Source: CAD feature listing. Evaluate the final solid. Frame: model axes, mm. A direction names the side the tool comes from. Give positions to 0.01 mm unless a question says otherwise; leave off trailing zeros. Write each loop counter-clockwise with the first axis right and the second up, starting at its lowest first coordinate (ties: lowest second). Pieces come first, ordered by that corner, then holes. Notation, with made-up numbers: (7.5, 18.25) -> (31.5, 18.25) arc R19 cw to (31.5, 55.25) -> close; hole circle Ø8 at (49.5, -5.5). An arc over 180 degrees is marked (long way). Write item = value, one per line.
from build123d import *

# Parameters (mm, degrees)
SKETCH1_W           = 12.7
SKETCH1_H           = 20.32
BOSS_EXTRUDE1_DEPTH = 3.175
SKETCH2_W           = 6.35
SKETCH2_H           = 3.175
CUT_EXTRUDE1_DEPTH  = 4.175
SKETCH3_R           = 1.27
CUT_EXTRUDE2_DEPTH  = 4.175


with BuildPart() as part:
    # Sketch1 → Boss-Extrude1 (new body)
    with BuildSketch(Plane(origin=(0, 0, 0), x_dir=(0, 0, -1), z_dir=(1, 0, 0))):
        Rectangle(SKETCH1_W, SKETCH1_H)
    extrude(amount=BOSS_EXTRUDE1_DEPTH)

    # Sketch2 → Cut-Extrude1 (cut, through all)
    with BuildSketch(Plane(origin=(3.175, 0, 0), x_dir=(0, 0, -1), z_dir=(1, 0, 0))):
        with Locations((0, -8.5725)):
            Rectangle(SKETCH2_W, SKETCH2_H)
    extrude(amount=-CUT_EXTRUDE1_DEPTH, mode=Mode.SUBTRACT)

    # Sketch3 → Cut-Extrude2 (cut, through all)
    with BuildSketch(Plane(origin=(3.175, 0, 0), x_dir=(0, 0, -1), z_dir=(1, 0, 0))):
        Circle(SKETCH3_R)
        with Locations((0, 7.62)):
            Circle(SKETCH3_R)
    extrude(amount=-CUT_EXTRUDE2_DEPTH, mode=Mode.SUBTRACT)


solid = part.part
1) Material intervals for L1, parallel to Y at x = 0.95, z = 0 (3 decimals); L2, parallel to Z at x = 2.9, y = -7.25 (3 decimals); L3, parallel to Y at x = 1.5, z = 0.75 (3 decimals), sorted ascending.
Computed:
L1 = -6.985 to -1.27, 1.27 to 6.35, 8.89 to 10.16
L2 = -6.35 to -3.175, 3.175 to 6.35
L3 = -6.985 to -1.025, 1.025 to 6.595, 8.645 to 10.16
2) Draft query along Y for faces 1 (the flat face through (0, 0, 2)), 2 (the cylindrical face through (1.61, 6.38, 0.28)), 3 (the flat face through (2, -6.985, 0)). Return one class per face: pulls with the +Y half, pulls with the -Y half, needs draft (parallel to the pull), parting line crosses it, or undercut.
Computed:
face_1 = needs draft
face_2 = undercut
face_3 = pulls with the -Y half
3) Cut plane A-A (y = 0). Return the cut outline in (x, z) (3 decimals), then the cut area to 3 significant figures.
Computed:
outline = (0, -6.35) -> (3.175, -6.35) -> (3.175, -1.27) -> (0, -1.27) -> close; (0, 1.27) -> (3.175, 1.27) -> (3.175, 6.35) -> (0, 6.35) -> close
area = 32.3 mm²
4) Cut plane B-B (z = 0). Return the cut outline in (x, y) (3 decimals).
Computed:
outline = (0, -6.985) -> (3.175, -6.985) -> (3.175, -1.27) -> (0, -1.27) -> close; (0, 1.27) -> (3.175, 1.27) -> (3.175, 6.35) -> (0, 6.35) -> close; (0, 8.89) -> (3.175, 8.89) -> (3.175, 10.16) -> (0, 10.16) -> close
5) Access query for faces 4 (the flat face through (2, -9, 3.175)), 5 (the flat face through (2, -10.16, -5)). Directions: +Z, -Z, +X, -X, +Y, -Y. A direction counts if a zero-diameter tool reaches every point of the face in a straight line with its end or side. Return the directions, or none.
Computed:
face_4 = +X, -X, -Y
face_5 = +Z, -Z, +X, -X, -Y
6) Cut plane D-D (z = -1.5). Return the cut outline in (x, y) (3 decimals).
Computed:
outline = (0, -6.985) -> (3.175, -6.985) -> (3.175, 10.16) -> (0, 10.16) -> close
7) Cut plane C-C (x = 2.35). Return the cut outline in (y, z) (3 decimals).
Computed:
outline = (-10.16, -6.35) -> (10.16, -6.35) -> (10.16, 6.35) -> (-10.16, 6.35) -> (-10.16, 3.175) -> (-6.985, 3.175) -> (-6.985, -3.175) -> (-10.16, -3.175) -> close; hole circle Ø2.54 at (0, 0); hole circle Ø2.54 at (7.62, 0)
8) Contact query for a flat-ended pin moving along its axis: pin 1 (1 mm diameter, centred on x = 2, z = -0.5, fed in from -Y) (3 decimals). Output: stop coordinate, or through.
Computed:
pin_1 = -6.985
